Could you check a few things on this model? Use its own coordinates, in mm. A direction names the side the tool comes from. Give positions to 0.01 mm unless a question says otherwise; leave off trailing zeros. Order: outer loops, then holes, each group sorted by start corner. A loop starts at its lowest first (then second) coordinate and runs counter-clockwise, first axis right, second up.
from build123d import *

# Parameters (mm, degrees)
SKETCH1_W           = 50.8
SKETCH1_H           = 38.1
BOSS_EXTRUDE1_DEPTH = 2.00000108
SKETCH2_W           = 2.00000108
SKETCH2_H           = 38.1
BOSS_EXTRUDE2_DEPTH = 38.1
SKETCH4_R           = 1.5875
CUT_EXTRUDE1_DEPTH  = 5.08
CUT_EXTRUDE3_DEPTH  = 2.54
FILLET1_R           = 3.175
SKETCH6_R           = 1.5875
CUT_EXTRUDE4_DEPTH  = 2.54


with BuildPart() as part:
    # Sketch1 → Boss-Extrude1 (new body)
    with BuildSketch(Plane(origin=(0, 0, 0), x_dir=(1, 0, 0), z_dir=(0, 1, 0))):
        with Locations((-21.481677668, -11.673311185)):
            Rectangle(SKETCH1_W, SKETCH1_H)
    extrude(amount=BOSS_EXTRUDE1_DEPTH)

    # Sketch2 → Boss-Extrude2 (add)
    with BuildSketch(Plane(origin=(0, 2.00000108, 0), x_dir=(1, 0, 0), z_dir=(0, 1, 0))):
        with Locations((-45.881677128, -11.673311185)):
            Rectangle(SKETCH2_W, SKETCH2_H)
    extrude(amount=BOSS_EXTRUDE2_DEPTH)

    # Sketch4 → Cut-Extrude1 (cut)
    with BuildSketch(Plane(origin=(0, 2.00000108, 0), x_dir=(1, 0, 0), z_dir=(0, 1, 0))):
        with Locations(Location((-0.844177668, -27.548311185, 0), (0, 0, 270))):
            Circle(SKETCH4_R)
        with Locations(Location((-7.194177668, -27.548311185, 0), (0, 0, 270))):
            Circle(SKETCH4_R)
        with Locations(Location((-13.544177668, -27.548311185, 0), (0, 0, 270))):
            Circle(SKETCH4_R)
        with Locations(Location((-19.894177668, -27.548311185, 0), (0, 0, 270))):
            Circle(SKETCH4_R)
        with Locations(Location((-26.244177668, -27.548311185, 0), (0, 0, 270))):
            Circle(SKETCH4_R)
        with Locations(Location((-32.594177668, -27.548311185, 0), (0, 0, 270))):
            Circle(SKETCH4_R)
        with Locations(Location((-38.944177668, -27.548311185, 0), (0, 0, 270))):
            Circle(SKETCH4_R)
        with Locations(Location((-0.844177668, 4.201688815, 0), (0, 0, 270))):
            Circle(SKETCH4_R)
        with Locations(Location((-7.194177668, 4.201688815, 0), (0, 0, 270))):
            Circle(SKETCH4_R)
        with Locations(Location((-13.544177668, 4.201688815, 0), (0, 0, 270))):
            Circle(SKETCH4_R)
        with Locations(Location((-19.894177668, 4.201688815, 0), (0, 0, 270))):
            Circle(SKETCH4_R)
        with Locations(Location((-26.244177668, 4.201688815, 0), (0, 0, 270))):
            Circle(SKETCH4_R)
        with Locations(Location((-32.594177668, 4.201688815, 0), (0, 0, 270))):
            Circle(SKETCH4_R)
        with Locations(Location((-38.944177668, 4.201688815, 0), (0, 0, 270))):
            Circle(SKETCH4_R)
    extrude(amount=-CUT_EXTRUDE1_DEPTH, mode=Mode.SUBTRACT)

    # Sketch5 → Cut-Extrude3 (cut)
    with BuildSketch(Plane(origin=(-46.881677668, 0, 30.723311185), x_dir=(0, 0, -1), z_dir=(1, 0, 0))):
        with BuildLine():
            ThreePointArc((19.05, 40.10000108), (32.520384182, 34.520385262), (38.1, 21.05000108))
            Line((38.1, 21.05000108), (38.1, 40.10000108))
            Line((38.1, 40.10000108), (19.05, 40.10000108))
        make_face()
        with BuildLine():
            Line((0, 40.10000108), (0, 21.05000108))
            ThreePointArc((0, 21.05000108), (5.579615818, 34.520385262), (19.05, 40.10000108))
            Line((19.05, 40.10000108), (0, 40.10000108))
        make_face()
    extrude(amount=CUT_EXTRUDE3_DEPTH, mode=Mode.SUBTRACT)

    # Fillet1
    fillet1_edges = [part.edges().sort_by_distance(p)[0] for p in [
        (-46.881677668, 0, 11.673311185),
        (-44.881676588, 2.00000108, 11.673311185),
        (3.918322332, 1.00000054, -7.376688815),
        (3.918322332, 1.00000054, 30.723311185),
    ]]
    fillet(fillet1_edges, radius=FILLET1_R)

    # Sketch6 → Cut-Extrude4 (cut)
    with BuildSketch(Plane(origin=(-46.881677668, 0, 30.723311185), x_dir=(0, 0, -1), z_dir=(1, 0, 0))):
        with Locations(Location((26.82875, 35.610695759, 0), (0, 0, 180))):
            Circle(SKETCH6_R)
        with Locations(Location((11.27125, 35.610695759, 0), (0, 0, 180))):
            Circle(SKETCH6_R)
        with Locations(Location((3.4925, 22.13750554, 0), (0, 0, 180))):
            Circle(SKETCH6_R)
        with BuildLine():
            Line((12.7, 21.05000108), (12.7, 15.525))
            ThreePointArc((12.7, 15.525), (19.05, 9.175), (25.4, 15.525))
            Line((25.4, 15.525), (25.4, 21.05000108))
            Line((25.4, 21.05000108), (25.4, 28.75001108))
            ThreePointArc((25.4, 28.75001108), (19.05, 35.10001108), (12.7, 28.75001108))
            Line((12.7, 28.75001108), (12.7, 21.05000108))
        make_face()
        with Locations(Location((34.6075, 22.13750554, 0), (0, 0, 180))):
            Circle(SKETCH6_R)
        with Locations(Location((26.82875, 8.664315321, 0), (0, 0, 180))):
            Circle(SKETCH6_R)
        with Locations(Location((11.27125, 8.664315321, 0), (0, 0, 180))):
            Circle(SKETCH6_R)
    extrude(amount=CUT_EXTRUDE4_DEPTH, mode=Mode.SUBTRACT)


solid = part.part
Item 1: Imagine slicing it at B-B on y = 33. List the corners of the cut face in (x, z) for me.
Findings:
outline: (-46.88, -3.16) - (-44.88, -3.16) - (-44.88, 6.96) - (-46.88, 6.96) - close; (-46.88, 16.39) - (-44.88, 16.39) - (-44.88, 26.51) - (-46.88, 26.51) - close
Item 2: We'd pull the mould along Z, two halves only. Please class faces 3 (the cylindrical face through (-0.367, 1.014, -2.687)), 4 (the flat face through (3.918, 1, 12)), 5 (the cylindrical face through (-45.896, 20.799, 28.084)): +Z half, -Z half, draft (parallel to the pull), parting line (faces both ways), or undercut.
Findings:
face 3: undercut
face 4: draft
face 5: undercut
Item 3: For pin 1 (5 mm diameter, centred on x = -0.84, z = -4.2, fed in from +Y); pin 2 (4 mm diameter, centred on x = -41.5, z = 24.5, fed in from +Y); pin 3 (5 mm diameter, centred on y = 8.66, z = 19.45, fed in from +X), each with a flat end and sliding along its axis, tell me the tip position at first contact or that it passes through.
Findings:
pin 1: stops at y = 2
pin 2: stops at y = 2.55
pin 3: stops at x = -44.88
Item 4: Imagine slicing it at D-D on z = 4. List the corners of the cut face in (x, y) for me (3 decimals), then the cut area to 3 significant figures.
Findings:
outline: (-46.882, 3.175) arc R3.175 ccw to (-43.707, 0) - (3.918, 0) - (3.918, 2) - (-41.707, 2) arc R3.175 cw to (-44.882, 5.175) - (-44.882, 7.08) - (-46.882, 7.08) - close; (-46.882, 10.248) - (-44.882, 10.248) - (-44.882, 34.027) - (-46.882, 34.027) - close; (-46.882, 37.195) - (-44.882, 37.195) - (-44.882, 38.486) - (-46.882, 38.486) - close
area: 162 mm2
Item 5: For faces 1 (the flat face through (-46, 22, 5.323)), 2 (the flat face through (-46.882, 21, 20)), which set-ups out of +Z, -Z, +X, -X, +Y, -Y let a thin tool reach every point of the face, with its end or its side?
Findings:
face 1: +X, -X
face 2: +Z, -Z, -X, +Y, -Y
Item 6: Imagine slicing it at C-C on x = -8. List the corners of the cut face in (y, z) for me.
Findings:
outline: (0, -7.38) - (2, -7.38) - (2, -5.57) - (0, -5.57) - close; (0, -2.83) - (2, -2.83) - (2, 26.18) - (0, 26.18) - close; (0, 28.92) - (2, 28.92) - (2, 30.72) - (0, 30.72) - close
Item 7: Please list where these lines run through material, in increasing order: line 1 along Y through (x, z) = (0, 6.5); line 2 along X through (y, z) = (38, 11).
Findings:
line 1: y = 0 to 2
line 2: x = -46.88 to -44.88
Item 8: Imagine slicing it at A-A on z = 15.5. List the corners of the cut face in (x, y) for me (3 decimals), then the cut area to 3 significant figures.
Findings:
outline: (-46.882, 3.175) arc R3.175 ccw to (-43.707, 0) - (3.918, 0) - (3.918, 2) - (-41.707, 2) arc R3.175 cw to (-44.882, 5.175) - (-44.882, 10.458) - (-46.882, 10.458) - close; (-46.882, 33.817) - (-44.882, 33.817) - (-44.882, 39.712) - (-46.882, 39.712) - close
area: 130 mm2
